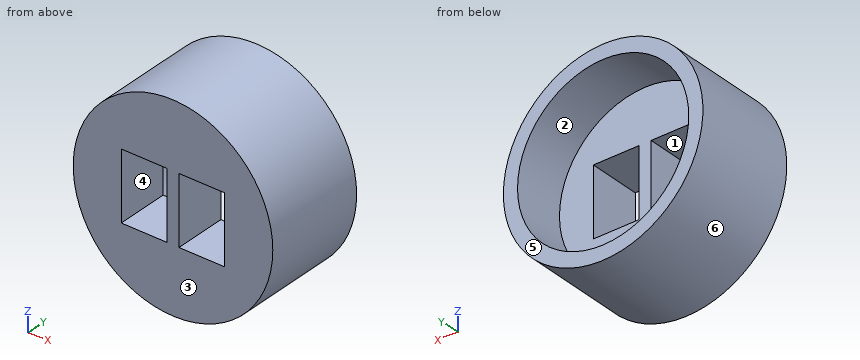
from build123d import *

# Parameters (mm, degrees)
SKETCH2_R           = 9.5
BOSS_EXTRUDE2_DEPTH = 10
SKETCH3_R           = 8.15
CUT_EXTRUDE1_DEPTH  = 5
SKETCH4_W           = 4.35
SKETCH4_H           = 6.5
CUT_EXTRUDE2_DEPTH  = 6


with BuildPart() as part:
    # Sketch2 → Boss-Extrude2 (new body)
    with BuildSketch(Plane(origin=(0, 0, 0), x_dir=(1, 0, 0), z_dir=(0, 1, 0))):
        Circle(SKETCH2_R)
    extrude(amount=BOSS_EXTRUDE2_DEPTH)

    # Sketch3 → Cut-Extrude1 (cut)
    with BuildSketch(Plane(origin=(0, 10, 0), x_dir=(1, 0, 0), z_dir=(0, 1, 0))):
        Circle(SKETCH3_R)
    extrude(amount=-CUT_EXTRUDE1_DEPTH, mode=Mode.SUBTRACT)

    # Sketch4 → Cut-Extrude2 (cut, through all)
    with BuildSketch(Plane(origin=(0, 5, 0), x_dir=(1, 0, 0), z_dir=(0, 1, 0))):
        with Locations((2.75, 0)):
            Rectangle(SKETCH4_W, SKETCH4_H)
        with Locations((-2.75, 0)):
            Rectangle(SKETCH4_W, SKETCH4_H)
    extrude(amount=-CUT_EXTRUDE2_DEPTH, mode=Mode.SUBTRACT)


solid = part.part
Can you work these out from the model? Positions are in its coordinate system, mm. Face numbers are marked on the shaded views. A direction names the side the tool comes from. Give positions to 0.01 mm unless a question says otherwise; leave off trailing zeros. Write each loop counter-clockwise with the first axis right and the second up, starting at its lowest first coordinate (ties: lowest second). Pieces come first, ordered by that corner, then holes. Notation, with made-up numbers: (-17.75, 45) -> (36.25, 45) arc R15 ccw to (36.25, 54) -> close; hole circle Ø8 at (52.5, 11). An arc over 180 degrees is marked (long way). Answer as a JSON object with one key per item and string values. Group by question number.
Item 1: Suppose I cut it at D-D (y = 8.5). Please give me the cut outline in (x, z).
Item 2: Please list where these lines run through material, in increasing order: line 1 (X direction, y = 9, z = 0); line 2 (X direction, y = 1.5, z = 1.75) (3 decimals); line 3 (X direction, y = 4, z = 1) (3 decimals). Write a range as [from, to].
Item 3: I'm going to push flat-ended pins straight in: P1, Ø8, axis at x = 2.5, z = -1.5, coming from the +Y side; P2, Ø3.5, axis at x = 3, y = 3.5, coming from the +Z side; P3, Ø2, axis at x = -2, y = 1.5, coming from the -Z side. Where does each tip first touch, or does it pass through?
Item 4: Suppose I cut it at C-C (x = 2). Please give me the cut outline in (y, z), plus the area to 3 significant figures.
Item 5: Suppose I cut it at A-A (z = 0). Please give me the cut outline in (x, y) (3 decimals).
Item 6: We'd pull the mould along X, two halves only. Please class the marked faces 4, 5 and 6: +X half, -X half, draft (parallel to the pull), parting line (faces both ways), or undercut.
Item 7: Suppose I cut it at B-B (x = 0). Please give me the cut outline in (y, z), plus the area to 4 significant figures.
Item 8: For the marked faces 1, 2 and 3, which set-ups out of +Z, -Z, +X, -X, +Y, -Y let a thin tool reach every point of the face, with its end or its side?
Findings:
{
 "1": {"outline": "circle Ø19 at (0, 0); hole circle Ø16.3 at (0, 0)"},
 "2": {"line 1": "x = [-9.5, -8.15], [8.15, 9.5]", "line 2": "x = [-9.337, -4.925], [-0.575, 0.575], [4.925, 9.337]", "line 3": "x = [-9.447, -4.925], [-0.575, 0.575], [4.925, 9.447]"},
 "3": {"P1": "stops at y = 5", "P2": "stops at z = 9.42", "P3": "stops at z = -9.45"},
 "4": {"outline": "(0, -9.29) -> (10, -9.29) -> (10, -7.9) -> (5, -7.9) -> (5, -3.25) -> (0, -3.25) -> close; (0, 3.25) -> (5, 3.25) -> (5, 7.9) -> (10, 7.9) -> (10, 9.29) -> (0, 9.29) -> close", "area": "74.2 mm²"},
 "5": {"outline": "(-9.5, 0) -> (-4.925, 0) -> (-4.925, 5) -> (-8.15, 5) -> (-8.15, 10) -> (-9.5, 10) -> close; (-0.575, 0) -> (0.575, 0) -> (0.575, 5) -> (-0.575, 5) -> close; (4.925, 0) -> (9.5, 0) -> (9.5, 10) -> (8.15, 10) -> (8.15, 5) -> (4.925, 5) -> close"},
 "6": {"face 4": "undercut", "face 5": "draft", "face 6": "parting line"},
 "7": {"outline": "(0, -9.5) -> (10, -9.5) -> (10, -8.15) -> (5, -8.15) -> (5, 8.15) -> (10, 8.15) -> (10, 9.5) -> (0, 9.5) -> close", "area": "108.5 mm²"},
 "8": {"face 1": "+Y, -Y", "face 2": "+Y", "face 3": "+Z, -Z, +X, -X, -Y"}
}
